Build history of the part. All positions in model axes, mm. A direction names the side the tool comes from. Round coordinates to 2 decimals unless told otherwise and drop trailing zeros. Write each loop counter-clockwise with the first axis right and the second up, starting at its lowest first coordinate (ties: lowest second). Pieces come first, ordered by that corner, then holes. Notation, with made-up numbers: M -36.5,28.5 L -2.5,28.5 A16 ccw -2.5,38.5 Z; hole C 74,38.5 d11. An arc over 180 degrees is marked long. Write item = value, one per line. Start each with the question number.
Q1. Band-saw the part on D-D on x = 12. Write the cut outline in (y, z), plus the area to 3 significant figures.
Q2. Pull direction X, two halves, no side cores. Call faces 3 (the flat face through (7, -23, 11)), 4 (the cylindrical face through (0, -30, 5)), 5 (the cylindrical face through (-24.722, -8.052, 5.423)), 6 (the cylindrical face through (-31, 9.76, 4.44)): released by +X, released by -X, zero draft, split by the parting line, or undercut.
Q3. Tool access for faces 1 (the cylindrical face through (24.63, -8.56, 5.42)), 2 (the flat face through (-13, -31, 9)): list every direction of +Z, -Z, +X, -X, +Y, -Y with a clear straight run to the whole face (end or side of a thin tool).
Q4. Band-saw the part on B-B on x = 0. Write the cut outline in (y, z).
Q5. Band-saw the part on A-A on y = 0. Write the cut outline in (x, z).
Q6. Drop flat-ended pins along their axis: P1, Ø2.5, axis at x = -26.63, y = -8.65, coming from the +Z side; P2, Ø4, axis at x = -14.5, y = 20.5, coming from the -Z side; P3, Ø4, axis at x = -21.5, z = 9, coming from the -Y side; P4, Ø5, axis at x = 25.5, y = -24.5, coming from the -Z side. Give the stop position or say it passes through.
Q7. Probe L1, parallel to Z at x = -31.5, y = -11; L2, parallel to Y at x = 8, z = 6.75; L3, parallel to X at y = 17, z = 8.5. List the from-to ranges inside material, lowest first.
Q8. Band-saw the part on C-C on z = 10. Write the cut outline in (x, y).
```python
from build123d import *

# Parameters (mm, degrees)
SKETCH_1_R          = 34.5
SKETCH_1_R_2        = 23
SKETCH_1_R_3        = 2
EXTRUDE_1_DEPTH     = 11
SKETCH_2_R          = 34.5
SKETCH_2_R_2        = 32.5
CUT_EXTRUDE_1_DEPTH = 9


with BuildPart() as part:
    # 草图1 → 凸台-拉伸1 (new body)
    with BuildSketch(Plane.XY):
        Circle(SKETCH_1_R)
        Circle(SKETCH_1_R_2, mode=Mode.SUBTRACT)
        with Locations((0, -28)):
            Circle(SKETCH_1_R_3, mode=Mode.SUBTRACT)
        with Locations((-26.629582456, -8.652475842)):
            Circle(SKETCH_1_R_3, mode=Mode.SUBTRACT)
        with Locations((-16.457987064, 22.652475842)):
            Circle(SKETCH_1_R_3, mode=Mode.SUBTRACT)
        with Locations((16.457987064, 22.652475842)):
            Circle(SKETCH_1_R_3, mode=Mode.SUBTRACT)
        with Locations((26.629582456, -8.652475842)):
            Circle(SKETCH_1_R_3, mode=Mode.SUBTRACT)
    extrude(amount=EXTRUDE_1_DEPTH)

    # 草图2 → 切除-拉伸1 (cut)
    with BuildSketch(Plane(origin=(0, 0, 0), x_dir=(-1, 0, 0), z_dir=(0, 0, -1))):
        Circle(SKETCH_2_R)
        Circle(SKETCH_2_R_2, mode=Mode.SUBTRACT)
    extrude(amount=-CUT_EXTRUDE_1_DEPTH, mode=Mode.SUBTRACT)


solid = part.part
```
Conclusion:
q1.outline = M -32.35,9 L -30.2,9 L -30.2,0 L -19.62,0 L -19.62,11 L -32.35,11 Z; M 19.62,0 L 30.2,0 L 30.2,9 L 32.35,9 L 32.35,11 L 19.62,11 Z
q1.area = 241 mm^2
q2.face_3 = zero draft
q2.face_4 = undercut
q2.face_5 = undercut
q2.face_6 = split by the parting line
q3.face_1 = +Z, -Z
q3.face_2 = -Z
q4.outline = M -34.5,9 L -32.5,9 L -32.5,0 L -30,0 L -30,11 L -34.5,11 Z; M -26,0 L -23,0 L -23,11 L -26,11 Z; M 23,0 L 32.5,0 L 32.5,9 L 34.5,9 L 34.5,11 L 23,11 Z
q5.outline = M -34.5,9 L -32.5,9 L -32.5,0 L -23,0 L -23,11 L -34.5,11 Z; M 23,0 L 32.5,0 L 32.5,9 L 34.5,9 L 34.5,11 L 23,11 Z
q6.P1 = through
q6.P2 = 0
q6.P3 = -28.46
q6.P4 = 9
q7.L1 = 9 to 11
q7.L2 = -31.5 to -21.56, 21.56 to 31.5
q7.L3 = -27.7 to -15.49, 15.49 to 27.7
q8.outline = C 0,0 d69; hole C -26.63,-8.65 d4; hole C 0,0 d46; hole C -16.46,22.65 d4; hole C 0,-28 d4; hole C 16.46,22.65 d4; hole C 26.63,-8.65 d4
